Verification items for the finished model (mm, model axes). Face numbers are marked on the shaded views. A direction names the side the tool comes from. Coordinates: 2 decimals unless noted, no trailing zeros. Write each loop counter-clockwise with the first axis right and the second up, starting at its lowest first coordinate (ties: lowest second). Pieces come first, ordered by that corner, then holes.
Autodesk Inventor part; units mm, degrees
ref_plane "YZ Plane" through (0, 0, 0) normal (1, 0, 0) x (0, 1, 0)
ref_plane "XZ Plane" through (0, 0, 0) normal (0, 1, 0) x (-1, 0, 0)
ref_plane "XY Plane" through (0, 0, 0) normal (0, 0, 1) x (1, 0, 0)
sketch "Boceto1" plane through (0, 0, 0) normal (0, 1, 0) x (-1, 0, 0)
  circle A0 centre (0, 0) radius 12.5
  dimension "d0" = 25
extrude "Extrusión1" add sketch "Boceto1" along normal blind 7.5 draft -5
sketch "Boceto2" plane through (0, 7.5, 0) normal (0, 1, 0) x (1, 0, 0)
  circle A0 centre (0, 0) radius 2.5
  dimension "d3" = 5
extrude "Extrusión2" cut sketch "Boceto2" against normal through all
sketch "Boceto3" plane through (0, 7.5, 0) normal (0, 1, 0) x (1, 0, 0)
  circle A0 centre (0, 0) radius 5
  dimension "d6" = 10
extrude "Extrusión3" cut sketch "Boceto3" against normal blind 5.2
fillet "Empalme1" radius 1 2 edges at (-5, 7.5, 0) (11.8438, 7.5, 0)
properties part number "RubberFoot"
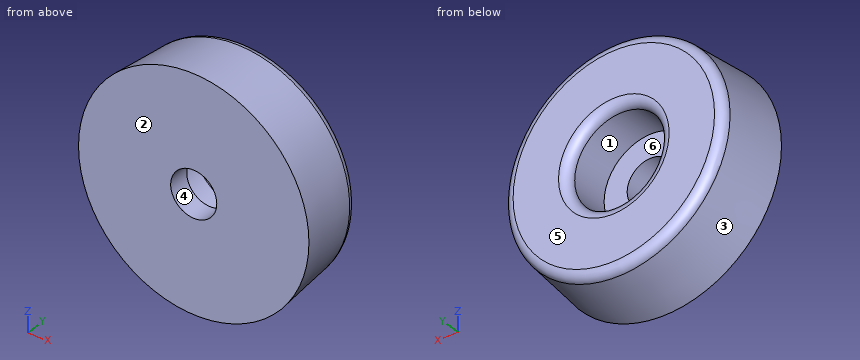
1. Sectioned sample at B-B, the plane x = 0. Record the boundary of the cut face in (y, z).
2. Tool access check on the marked faces 1 and 2. Record the directions out of +Z, -Z, +X, -X, +Y, -Y that give a thin tool (end or side, any length) a straight path to the whole face; none if there is none.
3. Sectioned sample at C-C, the plane y = 5.5. Record the boundary of the cut face in (x, z).
4. Material ranges on L1, parallel to Z at x = 0, y = 4.7; L2, parallel to Z at x = 4, y = 2.5; L3, parallel to X at y = 4, z = 3.75, recorded low to high.
5. Gauge pin test, flat ends, axial feed: P1, Ø5, axis at x = -1.5, z = 0.5, coming from the +Y side; P2, Ø1, axis at x = 2, y = 3, coming from the +Z side; P3, Ø4, axis at x = -1, z = -3, coming from the +Y side. Record the tip position at first contact, or that the pin passes through.
6. Sectioned sample at A-A, the plane z = 0. Record the boundary of the cut face in (x, y).
7. Draft check along X on the marked faces 3, 4, 5 and 6. Enter one of: pulls with the +X half, pulls with the -X half, needs draft (parallel to the pull), parting line crosses it, or undercut.
8. Sectioned sample at D-D, the plane y = 1.75. Record the boundary of the cut face in (x, z).
Outcome:
1. outline: (0, -12.5) - (6.59, -11.92) arc R1 ccw to (7.5, -10.93) - (7.5, -6) arc R1 ccw to (6.5, -5) - (2.3, -5) - (2.3, -2.5) - (0, -2.5) - close; (0, 2.5) - (2.3, 2.5) - (2.3, 5) - (6.5, 5) arc R1 ccw to (7.5, 6) - (7.5, 10.93) arc R1 ccw to (6.59, 11.92) - (0, 12.5) - close
2. face 1: +Y
2. face 2: +Z, -Z, +X, -X, -Y
3. outline: circle Ø24.04 at (0, 0); hole circle Ø10 at (0, 0)
4. L1: z = -12.09 to -5, 5 to 12.09
4. L2: z = -11.61 to -3, 3 to 11.61
4. L3: x = -11.56 to -3.31, 3.31 to 11.56
5. P1: stops at y = 2.3
5. P2: stops at z = 12.16
5. P3: stops at y = 7.05
6. outline: (-12.5, 0) - (-2.5, 0) - (-2.5, 2.3) - (-5, 2.3) - (-5, 6.5) arc R1 ccw to (-6, 7.5) - (-10.93, 7.5) arc R1 ccw to (-11.92, 6.59) - close; (2.5, 0) - (12.5, 0) - (11.92, 6.59) arc R1 ccw to (10.93, 7.5) - (6, 7.5) arc R1 ccw to (5, 6.5) - (5, 2.3) - (2.5, 2.3) - close
7. face 3: parting line crosses it
7. face 4: undercut
7. face 5: needs draft
7. face 6: undercut
8. outline: circle Ø24.69 at (0, 0); hole circle Ø5 at (0, 0)
